Verification items for the finished model (mm, model axes). Give positions to 0.01 mm unless a question says otherwise; leave off trailing zeros. Write each loop counter-clockwise with the first axis right and the second up, starting at its lowest first coordinate (ties: lowest second). Pieces come first, ordered by that corner, then holes. Notation, with made-up numbers: (39.25, 18.25) - (66.25, 18.25) arc R11 cw to (66.25, 38.25) - close; hole circle Ø2 at (27.5, 69). An arc over 180 degrees is marked (long way). Put each result on its own line as item: value.
from build123d import *

# Parameters (mm, degrees)
F1_DEPTH = 25
F2_R     = 2
F3_R     = 8


with BuildPart() as f1:
    # F0 (on Top) → F1 (new body)
    with BuildSketch(Plane.XY):
        with BuildLine():
            Line((-54.407789, -23.747728), (66.092211, -23.747728))
            Line((66.092211, -23.747728), (66.092211, -4.747728))
            ThreePointArc((66.092211, -4.747728), (44.589047, 6.797961), (20.592211, 11.252272))
            Line((20.592211, 11.252272), (-54.407789, 11.252272))
            Line((-54.407789, 11.252272), (-54.407789, -23.747728))
        make_face()
    extrude(amount=F1_DEPTH)

    # F2
    f2_edges = [f1.edges().sort_by_distance(p)[0] for p in [
        (-54.407789, -23.747728, 12.5),
        (66.092211, -23.747728, 12.5),
        (-54.407789, 11.252272, 12.5),
    ]]
    fillet(f2_edges, radius=F2_R)

    # F3
    f3_edges = [f1.edges().sort_by_distance(p)[0] for p in [
        (66.092211, -4.747728, 12.5),
    ]]
    fillet(f3_edges, radius=F3_R)


solid = f1.part
Q1. Release check for a two-part mould opening along Y. For faces 1 (the face through (65.18, -5.15, 12.68)), 2 (the face through (5, -6, 25)), 3 (the face through (-53.806, -23.177, 12.675)) record: released by +Y, released by -Y, zero draft, split by the parting line, or undercut.
Answers follow:
face 1: released by +Y
face 2: zero draft
face 3: released by -Y
Q2. Scan lines: line 1 along X through (y, z) = (-22, 21.5); line 2 along Y through (x, z) = (36, 11.5); line 3 along Y through (x, z) = (60, 21.25). Record each from-to range of solid material in increasing order.
Answers follow:
line 1: x = -54.39 to 66.08
line 2: y = -23.75 to 9.28
line 3: y = -23.75 to -0.57
Q3. Section check B-B, the plane x = 47. Record the cut outline in (y, z).
Answers follow:
outline: (-23.75, 0) - (5.91, 0) - (5.91, 25) - (-23.75, 25) - close
Q4. Section check C-C, the plane y = 5.5. Record the cut outline in (x, z).
Answers follow:
outline: (-54.41, 0) - (48.02, 0) - (48.02, 25) - (-54.41, 25) - close
Q5. Section check A-A, the plane z = 10.25. Record the cut outline in (x, y), plus the area to 3 significant figures.
Answers follow:
outline: (-54.41, -21.75) arc R2 ccw to (-52.41, -23.75) - (64.09, -23.75) arc R2 ccw to (66.09, -21.75) - (66.09, -8.86) arc R8 ccw to (62.56, -2.23) arc R79.25 ccw to (20.59, 11.25) - (-52.41, 11.25) arc R2 ccw to (-54.41, 9.25) - close
area: 3,970 mm2
Q6. Go/stop test with a flat-tipped pin: pin 1 Ø1.5 at (x, y) = (50.5, -0.5) entering from -Z. Record where the tip stops, or that it passes through.
Answers follow:
pin 1: stops at z = 0
